```python
from build123d import *

# Parameters (mm, degrees)
BOSS_EXTRUDE1_DEPTH     = 10
SKETCH2_W               = 18
SKETCH2_H               = 7.18
CUT_EXTRUDE1_DEPTH      = 4.5
CUT_EXTRUDE1_DEPTH_BACK = 10
SKETCH3_R               = 2.5
CUT_EXTRUDE2_DEPTH      = 11
SKETCH4_R               = 2.5
CUT_EXTRUDE3_DEPTH      = 11
SKETCH5_W               = 40.184042348
SKETCH5_H               = 7.210208874
CUT_EXTRUDE4_DEPTH      = 10


with BuildPart() as part:
    # Sketch1 → Boss-Extrude1 (new body)
    with BuildSketch(Plane(origin=(0, 0, 0), x_dir=(1, 0, 0), z_dir=(0, 1, 0))):
        with BuildLine():
            Line((4.5, 0), (4.5, -6.46875))
            Line((4.5, -6.46875), (-6.330925138, -24.986801467))
            ThreePointArc((-6.330925138, -24.986801467), (-12.518133398, -24.960664715), (-9.416959682, -19.606698823))
            Line((-9.416959682, -19.606698823), (-0.560766754, -4.464923364))
            ThreePointArc((-0.560766754, -4.464923364), (-2.977125258, 3.374422202), (4.5, 0))
        make_face()
    extrude(amount=BOSS_EXTRUDE1_DEPTH)

    # Sketch2 → Cut-Extrude1 (cut, two sides)
    with BuildSketch(Plane.XY) as cut_extrude1_sk:
        with Locations((4.5, 5)):
            Rectangle(SKETCH2_W, SKETCH2_H)
    extrude(amount=CUT_EXTRUDE1_DEPTH, mode=Mode.SUBTRACT)
    extrude(cut_extrude1_sk.sketch, amount=-CUT_EXTRUDE1_DEPTH_BACK, mode=Mode.SUBTRACT)

    # Sketch3 → Cut-Extrude2 (cut, through all)
    with BuildSketch(Plane(origin=(0, 10, 0), x_dir=(1, 0, 0), z_dir=(0, 1, 0))):
        Circle(SKETCH3_R)
    extrude(amount=-CUT_EXTRUDE2_DEPTH, mode=Mode.SUBTRACT)

    # Sketch4 → Cut-Extrude3 (cut, through all)
    with BuildSketch(Plane(origin=(0, 10, 0), x_dir=(1, 0, 0), z_dir=(0, 1, 0))):
        with Locations((-9.416959682, -23.181827052)):
            Circle(SKETCH4_R)
    extrude(amount=-CUT_EXTRUDE3_DEPTH, mode=Mode.SUBTRACT)

    # Sketch5 → Cut-Extrude4 (cut)
    with BuildSketch(Plane(origin=(6.172069089, 0, 3.609948831), x_dir=(0.50486984, 0, -0.863195485), z_dir=(0.863195485, 0, 0.50486984))):
        with Locations((-1.612465403, 5)):
            Rectangle(SKETCH5_W, SKETCH5_H)
    extrude(amount=-CUT_EXTRUDE4_DEPTH, mode=Mode.SUBTRACT)


solid = part.part
```
Model file for the job. Use its own axes, mm. A direction names the side the tool comes from. Give positions to 0.01 mm unless a question says otherwise; leave off trailing zeros. Order: outer loops, then holes, each group sorted by start corner. A loop starts at its lowest first (then second) coordinate and runs counter-clockwise, first axis right, second up.
1) Mould opens along Y. For faces 3 (the flat face through (-2, 10, 10)), 4 (the flat face through (-7.094, 4.95, 20.995)), 5 (the cylindrical face through (-0.54, 9.31, 2.44)) say: +Y half, -Y half, draft (parallel to the pull), parting line (faces both ways), or undercut.
2) Pin check, flat tips, straight feed: pin 1 (6 mm diameter, centred on y = 8.5, z = 11, fed in from -X); pin 2 (4 mm diameter, centred on y = 3.5, z = 18, fed in from -X); pin 3 (2 mm diameter, centred on y = 9, z = 7.5, fed in from -X). Stop position of each tip, or through.
3) Wall check: probe 1 along Y at (x, z) = (1.5, 3); probe 2 along X at (y, z) = (8.9, 0); probe 3 along Z at (x, y) = (0, 0.4). Give the ranges that are in metal, low to high.
4) Saw through at C-C, the plane x = -11. Write the cut outline in (y, z).
5) Saw through at D-D, the plane y = 0.5. Write the cut outline in (x, z), then the cut area to 3 significant figures.
6) Saw through at A-A, the plane z = 7.5. Write the cut outline in (x, y), then the cut area to 3 significant figures.
7) Saw through at B-B, the plane x = 2. Write the cut outline in (y, z).
8) 3-axis set-ups, long thin cutter, end or side, ignore diameter. For faces 1 (the flat face through (-3, 1.41, -1)), 2 (the flat face through (-5.05, 9.29, 12.14)): which of +Z, -Z, +X, -X, +Y, -Y reach the whole face in a straight line?
Computed:
1. face 3: +Y half
1. face 4: undercut
1. face 5: draft
2. pin 1: stops at x = -6.14
2. pin 2: stops at x = -11.05
2. pin 3: stops at x = -2.92
3. probe 1: y = 0 to 1.39, 8.61 to 10
3. probe 2: x = -4.5 to -2.5, 2.5 to 4.5
3. probe 3: z = -4.5 to -2.5, 2.5 to 14.16
4. outline: (0, 19.98) - (10, 19.98) - (10, 21.25) - (0, 21.25) - close; (0, 25.12) - (10, 25.12) - (10, 26.39) - (0, 26.39) - close
5. outline: (-9.42, 19.61) - (-0.56, 4.46) arc R4.5 ccw (long way) to (4.5, 0) - (4.5, 6.47) - (-6.33, 24.99) arc R3.58 ccw (long way) to start; hole circle Ø5 at (-9.42, 23.18); hole circle Ø5 at (0, 0)
5. area: 171 mm2
6. outline: (-2.34, 0) - (3.9, 0) - (3.9, 1.39) - (-2.34, 1.39) - close; (-2.34, 8.61) - (3.9, 8.61) - (3.9, 10) - (-2.34, 10) - close
6. area: 17.4 mm2
7. outline: (0, -4.03) - (1.39, -4.03) - (1.39, -1.5) - (0, -1.5) - close; (0, 1.5) - (1.39, 1.5) - (1.39, 10.74) - (0, 10.74) - close; (8.61, -4.03) - (10, -4.03) - (10, -1.5) - (8.61, -1.5) - close; (8.61, 1.5) - (10, 1.5) - (10, 10.74) - (8.61, 10.74) - close
8. face 1: +Z, -Z, +X, -X
8. face 2: -X, +Y, -Y
